Here's how the part is built. I have some questions about the finished solid (model axes, mm). A direction names the side the tool comes from. Round coordinates to 2 decimals unless told otherwise and drop trailing zeros. Loops run counter-clockwise (first coordinate to the right, second up) from the corner with the lowest first, then second, coordinate; pieces in that order, holes last. Notation, with made-up numbers: (83, 15) - (114, 15) arc R13 ccw to (114, 19) - close; hole circle Ø1 at (88, 44.5). An arc over 180 degrees is marked (long way). Answer as a JSON object with one key per item and string values. Group by question number.
1) I want a section at B-B, the plane x = 22. Please give me the cut outline in (y, z), then the cut area to 3 significant figures.
2) If we mould it in two halves opening along Z, with no side actions, what happens to faces 4 (the face through (12.91, 39.24, 2.21)), 5 (the face through (20.1, 41.1, 3.7)), 6 (the face through (30.919, 40.957, 0.79)), 7 (the face through (10.757, 40.957, 1.72))? For each: pulls with the +Z half, pulls with the -Z half, needs draft (parallel to the pull), parting line crosses it, or undercut.
3) I want a section at A-A, the plane z = 16.5. Please give me the cut outline in (x, y).
4) If I drill on line 1 along X through (y, z) = (40, 16.5); line 2 along Z through (x, y) = (12.5, 40.35), over which ranges is the centre line in solid material (lowest first)? Write a range as [from, to].
5) Which directions (+Z, -Z, +X, -X, +Y, -Y) give clear straight access to the entire face, cutting with the end or side of a thin tool? Please do faces 1 (the face through (30.8, 40, 19)), 2 (the face through (13.081, 39.243, 0.79)), 3 (the face through (12.78, 40.09, 0.7)).
from build123d import *

# Parameters (mm, degrees)
BOX026_W               = 2
BOX026_H               = 2
BOX026_DEPTH           = 4
BOX026_PLACEMENT_ANGLE = 45
BOX027_W               = 2
BOX027_H               = 2
BOX027_DEPTH           = 4
BOX027_PLACEMENT_ANGLE = 45
BOX025_W               = 17.6
BOX025_H               = 2
BOX025_DEPTH           = 12.85
CYLINDER063_R          = 8.8
CYLINDER063_DEPTH      = 2
BOX024_W               = 25.5
BOX024_H               = 2
BOX024_DEPTH           = 26
FILLET_R               = 0.5


with BuildPart() as obj1:
    # Box026 → Box026 (new body)
    with BuildSketch(Plane.XY):
        with Locations((1, 1)):
            Rectangle(BOX026_W, BOX026_H)
    extrude(amount=BOX026_DEPTH)


with BuildPart() as obj1_1:
    # Box026 placement: moved
    add(obj1.part.moved(Location((-12.75, 0, -13.15))).rotate(Axis((-12.75, 0, -13.15), (0, 1, 0)), BOX026_PLACEMENT_ANGLE))


with BuildPart() as obj2:
    # Part__Mirroring006: instance of obj1
    add(obj1_1.part.mirror(Plane(origin=(0, 0, 0), x_dir=(0, -1, 0), z_dir=(1, 0, 0))))


with BuildPart() as obj3:
    # Box027 → Box027 (new body)
    with BuildSketch(Plane.XY):
        with Locations((1, 1)):
            Rectangle(BOX027_W, BOX027_H)
    extrude(amount=BOX027_DEPTH)


with BuildPart() as obj3_1:
    # Box027 placement: moved
    add(obj3.part.moved(Location((-12.75, 0, -13.15))).rotate(Axis((-12.75, 0, -13.15), (0, 1, 0)), BOX027_PLACEMENT_ANGLE))


with BuildPart() as obj4:
    # Box025 → Box025 (new body)
    with BuildSketch(Plane(origin=(-8.8, 0, 0), x_dir=(1, 0, 0), z_dir=(0, 0, 1))):
        with Locations((8.8, 1)):
            Rectangle(BOX025_W, BOX025_H)
    extrude(amount=BOX025_DEPTH)


with BuildPart() as obj5:
    # Cylinder063 → Cylinder063 (new body)
    with BuildSketch(Plane(origin=(0, 0, 0), x_dir=(1, 0, 0), z_dir=(0, 1, 0))):
        Circle(CYLINDER063_R)
    extrude(amount=CYLINDER063_DEPTH)

    # Fusion062: union obj2, obj3, obj4
    add(obj2.part)
    add(obj3_1.part)
    add(obj4.part)


with BuildPart() as toplevelpart_outletkey:
    # Box024 → Box024 (new body)
    with BuildSketch(Plane(origin=(-12.75, 0, -13.15), x_dir=(1, 0, 0), z_dir=(0, 0, 1))):
        with Locations((12.75, 1)):
            Rectangle(BOX024_W, BOX024_H)
    extrude(amount=BOX024_DEPTH)

    # Cut021: cut obj5
    add(obj5.part, mode=Mode.SUBTRACT)

    # Fillet
    fillet_edges = [toplevelpart_outletkey.edges().sort_by_distance(p)[0] for p in [
        (-12.75, 0, -0.15),
        (-12.75, 2, -0.15),
        (-11.335786, 0, -11.735786),
        (-9.214466, 0, -11.02868),
        (-9.214466, 0, -12.442893),
        (0, 0, -13.15),
        (9.214466, 0, -12.442893),
        (9.214466, 0, -11.02868),
        (11.335786, 0, -11.735786),
        (12.75, 0, -0.15),
        (10.775, 0, 12.85),
        (8.8, 0, 6.425),
        (0, 0, -8.8),
        (-8.8, 0, 6.425),
        (-10.775, 0, 12.85),
        (-10.775, 2, 12.85),
        (-11.335786, 2, -11.735786),
        (-9.214466, 2, -11.02868),
        (-9.214466, 2, -12.442893),
        (0, 2, -13.15),
        (9.214466, 2, -12.442893),
        (9.214466, 2, -11.02868),
        (11.335786, 2, -11.735786),
        (12.75, 2, -0.15),
        (10.775, 2, 12.85),
        (8.8, 2, 6.425),
        (0, 2, -8.8),
        (-8.8, 2, 6.425),
    ]]
    fillet(fillet_edges, radius=FILLET_R)


with BuildPart() as toplevelpart_outletkey_1:
    # Fillet placement: moved
    add(toplevelpart_outletkey.part.moved(Location((22, 39.1, 13.15))))


solid = toplevelpart_outletkey_1.part
Outcome:
{
 "1": {"outline": "(39.1, 0.5) arc R0.5 ccw to (39.6, 0) - (40.6, 0) arc R0.5 ccw to (41.1, 0.5) - (41.1, 3.85) arc R0.5 ccw to (40.6, 4.35) - (39.6, 4.35) arc R0.5 ccw to (39.1, 3.85) - close", "area": "8.49 mm^2"},
 "2": {"face 4": "undercut", "face 5": "needs draft", "face 6": "undercut", "face 7": "pulls with the -Z half"},
 "3": {"outline": "(9.25, 39.6) arc R0.5 ccw to (9.75, 39.1) - (12.7, 39.1) arc R0.5 ccw to (13.2, 39.6) - (13.2, 40.6) arc R0.5 ccw to (12.7, 41.1) - (9.75, 41.1) arc R0.5 ccw to (9.25, 40.6) - close; (30.8, 39.6) arc R0.5 ccw to (31.3, 39.1) - (34.25, 39.1) arc R0.5 ccw to (34.75, 39.6) - (34.75, 40.6) arc R0.5 ccw to (34.25, 41.1) - (31.3, 41.1) arc R0.5 ccw to (30.8, 40.6) - close"},
 "4": {"line 1": "[9.25, 13.2], [30.8, 34.75]", "line 2": "[0, 0.42], [2.41, 26]"},
 "5": {"face 1": "+Z, +Y, -Y", "face 2": "-Y", "face 3": "+Y, -Y"}
}
